Design review of the part built by this model. Coordinates are the model's own, in mm. A direction names the side the tool comes from. Coordinates: 2 decimals unless noted, no trailing zeros. Write each loop counter-clockwise with the first axis right and the second up, starting at its lowest first coordinate (ties: lowest second). Pieces come first, ordered by that corner, then holes.
```python
from build123d import *

# Parameters (mm, degrees)
SKETCH1_W = 1
SKETCH1_H = 1


with BuildPart() as part:
    # Sketch1 → Revolve1 (revolve)
    with BuildSketch(Plane.XY, mode=Mode.PRIVATE) as revolve1_sk:
        with BuildLine():
            Line((-70, 26), (-70, 0))
            ThreePointArc((-70, 0), (-49.497474683, -49.497474683), (0, -70))
            Line((0, -70), (0, -69))
            ThreePointArc((0, -69), (-48.790367902, -48.790367902), (-69, 0))
            Line((-69, 0), (-69, 22))
            Line((-69, 22), (-62.585786438, 22))
            Line((-62.585786438, 22), (-59.292893219, 25.292893219))
            Line((-59.292893219, 25.292893219), (-59.292893219, 27))
            Line((-59.292893219, 27), (-60.171572875, 27))
            ThreePointArc((-60.171572875, 27), (-60.043204321, 26.507305936), (-60, 26))
            Line((-60, 26), (-63, 23))
            Line((-63, 23), (-69, 23))
            Line((-69, 23), (-69, 26))
            Line((-69, 26), (-70, 26))
        make_face()
        with Locations((-69.5, 26.5)):
            Rectangle(SKETCH1_W, SKETCH1_H)
        with BuildLine():
            ThreePointArc((-67, 30), (-69.121320344, 29.121320344), (-70, 27))
            Line((-70, 27), (-69, 27))
            ThreePointArc((-69, 27), (-68.414213562, 28.414213562), (-67, 29))
            Line((-67, 29), (-63, 29))
            ThreePointArc((-63, 29), (-61.267949192, 28.449489743), (-60.171572875, 27))
            Line((-60.171572875, 27), (-59.292893219, 27))
            ThreePointArc((-59.292893219, 27), (-60.171572875, 29.121320344), (-62.292893219, 30))
            Line((-62.292893219, 30), (-67, 30))
        make_face()
    revolve(revolve1_sk.sketch.rotate(Axis((0, 64.231283711, 0), (0, -1, 0)), 270), axis=Axis((0, 64.231283711, 0), (0, -1, 0)))


solid = part.part
```
(1) Consider section A-A (y = -46.5). Give the boundary of the cut face in (x, z).
(2) Consider section B-B (z = -9). State how many separate pieces and enclosed holes the cut face has, plus the area to 3 significant figures.
(3) Insertion check: pin 1 Ø5 at (y, z) = (-16, 51.5) entering from +X; pin 2 Ø12 at (x, y) = (-54.5, -4.5) entering from +Z; pin 3 Ø2 at (x, y) = (31.5, -33) entering from +Z. Each pin has a flat end and moves straight along its axis. Give the tip position at first contact, or say it passes through.
(4) Wall thickness on line 1 (X direction, y = 5.75, z = 0); line 2 (Y direction, x = 54, z = -27.5); line 3 (X direction, y = 26.35, z = 0): over which ranges is each line inside the solid? List them lowest first.
(5) For faces 4 (the cylindrical face through (-17.81, 26.158, 56.555)), 5 (the flat face through (44.4, 29, -45)), list the 3-axis set-ups (+Z, -Z, +X, -X, +Y, -Y) from which the entire face can be reached by the end or side of a thin tool; tool diameter is ignored.
(6) Mouldability with a two-part tool opening along Z and no side actions: class faces 1 (the flat face through (44.4, 30, -44.4)), 2 (the cylindrical face through (42.594, 13.311, -55.55)), 3 (the conical face through (23.05, 25.81, 55.6)) as +Z half, -Z half, draft (parallel to the pull), parting line (faces both ways), or undercut.
Results:
1. outline: circle Ø104.65 at (0, 0); hole circle Ø101.96 at (0, 0)
2. separate pieces: 1
2. enclosed holes: 2
2. area: 323 mm2
3. pin 1: stops at x = 47.49
3. pin 2: stops at z = 50.3
3. pin 3: stops at z = 53.94
4. line 1: x = -70 to -69, 69 to 70
4. line 2: y = -35.04 to -33, 23.99 to 25.4, 27.8 to 29.48
4. line 3: x = -70 to -69, -60.02 to -59.29, 59.29 to 60.02, 69 to 70
5. face 4: +Y
5. face 5: none
6. face 1: draft
6. face 2: parting line
6. face 3: undercut
